Autodesk Inventor part; units mm, degrees
ref_plane "YZ Plane" through (0, 0, 0) normal (1, 0, 0) x (0, 1, 0)
ref_plane "XZ Plane" through (0, 0, 0) normal (0, 1, 0) x (-1, 0, 0)
ref_plane "XY Plane" through (0, 0, 0) normal (0, 0, 1) x (1, 0, 0)
sketch "Sketch1" plane through (0, 0, 0) normal (0, 0, 1) x (1, 0, 0)
  line L0 (-32.3906, 7.996) -> (-32.3906, -0.004) construction
  line L1 (-40.3906, -0.004) -> (-32.3906, -0.004) construction
  line L2 (61.6987, -0.004) -> (-73.3826, -0.004) construction
  line L3 (24.6094, 8.046) -> (24.6094, 6.796)
  line L4 (-40.3906, -0.004) -> (-39.1406, -0.004)
  line L5 (21.2094, 9.588) -> (21.2094, 3.996) construction
  line L6 (24.6094, 6.796) -> (21.4757, 6.7961)
  line L7 (24.6094, 8.046) -> (-20.3906, 8.046)
  line L8 (-40.3906, -0.004) -> (-40.3906, 3.996)
  arc A0 (-20.3906, 8.046) -> (-40.3906, 3.996) centre (-20.3906, -43.3617) ccw
  line L9 (20.9432, 6.7961) -> (-22.0568, 6.7961)
  line L10 (-39.1406, -0.004) -> (-39.1406, 2.996)
  arc A1 (-22.0568, 6.7961) -> (-39.1406, 2.996) centre (-20.84, -38.9748) ccw
  line L11 (20.9432, 6.7961) -> (21.4757, 6.7961)
  point P0 (0, 0)
  point P1 (-32.3906, 6.746)
  dimension "d3" = 1.25
  dimension "d4" = 65
  dimension "d6" = 6.8
  dimension "d7" = 8.05
  dimension "d8" = 3.4
  dimension "d12" = 45
  dimension "d13" = 4
  dimension "d14" = 3
  dimension "d16" = 43
revolve "Revolution1" add sketch "Sketch1" angle 360 about axis through (61.6987, -0.004, 0) along (-1, 0, 0)
fillet "Fillet1" radius 0.2 1 edges at (24.6094, -8.054, 0)
fillet "Fillet2" radius 5.7 1 edges at (-40.3906, -4.004, 0)
fillet "Fillet3" radius 3.9 1 edges at (-39.1406, -3.004, 0)
properties part number "Cap"
Verification items for the finished model (mm, model axes). Coordinates: 2 decimals unless noted, no trailing zeros. Order: outer loops, then holes, each group sorted by start corner. A loop starts at its lowest first (then second) coordinate and runs counter-clockwise, first axis right, second up. Notation, with made-up numbers: (83, -30) - (107, -30) arc R29 cw to (107, -2) - close; hole circle Ø10 at (52, -13). An arc over 180 degrees is marked (long way). Return JSON: item names as keys, results as strings.
(1) Thickness scan on line 1 along Y through (x, z) = (22.4, 0); line 2 along Z through (x, y) = (-23, -3.25); line 3 along Y through (x, z) = (-31, 1.25). Record the ranges inside material, lowest first.
Filled sheet:
{"line 1": "y = -8.05 to -6.8, 6.8 to 8.05", "line 2": "z = -7.29 to -5.94, 5.94 to 7.29", "line 3": "y = -6.83 to -5.54, 5.53 to 6.83"}
(2) Mould release check, pull along Y, two halves, no side actions. Record for faces 1 (the flat face through (24.609, -6, -4)), 2 (the cylindrical face through (23.021, -1.478, 6.638)), 3 (the cylindrical face through (1.7, -1.75, 7.86)): pulls with the +Y half, pulls with the -Y half, needs draft (parallel to the pull), parting line crosses it, or undercut.
Filled sheet:
{"face 1": "needs draft", "face 2": "undercut", "face 3": "parting line crosses it"}
(3) Go/stop test with flat-tipped pins: pin 1 (1 mm diameter, centred on x = -7.5, y = -3.5, fed in from +Z); pin 2 (0.8 mm diameter, centred on y = 0, z = 0, fed in from +X); pin 3 (2 mm diameter, centred on x = -27, z = -0.5, fed in from +Y). Record where each tip stops, or that it passes through.
Filled sheet:
{"pin 1": "stops at z = 7.47", "pin 2": "stops at x = -39.14", "pin 3": "stops at y = 7.73"}
(4) Section check A-A, the plane x = 10.5. Record the cut outline in (y, z), and give its area (3 significant figures).
Filled sheet:
{"outline": "circle Ø16.1 at (0, 0); hole circle Ø13.6 at (0, 0)", "area": "58.3 mm^2"}
